from build123d import *

# Parameters (mm, degrees)
SKETCH1_W           = 27.7876
SKETCH1_H           = 4.572
CUT_EXTRUDE1_DEPTH  = 40.562666891
CUT_EXTRUDE2_DEPTH  = 40.562666891
CUT_EXTRUDE3_DEPTH  = 40.562666891
CUT_EXTRUDE4_DEPTH  = 40.562666891
CUT_EXTRUDE5_DEPTH  = 40.530803878
CUT_EXTRUDE6_DEPTH  = 40.530803878
SKETCH8_R           = 14.2875
BOSS_EXTRUDE1_DEPTH = 0.889
SKETCH9_R           = 12.9794
BOSS_EXTRUDE2_DEPTH = 0.8128
BOSS_EXTRUDE2_TAPER = 45
SKETCH10_R          = 12.1666
BOSS_EXTRUDE3_DEPTH = 18.2372
BOSS_EXTRUDE4_START = 0.889
SKETCH11_R          = 14.2875
BOSS_EXTRUDE4_DEPTH = 0.889
CUT_EXTRUDE7_DEPTH  = 47.764743892
SKETCH13_W          = 2.5908
SKETCH13_H          = 4.572
SKETCH14_W          = 2.5908
SKETCH14_H          = 4.572
SKETCH15_W          = 2.5908
SKETCH15_H          = 4.572
SKETCH16_W          = 2.5908
SKETCH16_H          = 4.572
SKETCH17_W          = 2.5908
SKETCH17_H          = 4.572
SKETCH18_W          = 2.5908
SKETCH18_H          = 4.572
CHAMFER1_SIZE       = 0.254
FILLET1_R           = 0.127
FILLET2_R           = 0.7874
SKETCH19_R          = 9.350419414
BOSS_EXTRUDE7_DEPTH = 25.4


with BuildPart() as part:
    # Sketch1 → Revolve1 (revolve)
    with BuildSketch(Plane.XY, mode=Mode.PRIVATE) as revolve1_sk:
        with Locations((13.8938, 3.175)):
            Rectangle(SKETCH1_W, SKETCH1_H)
    revolve(revolve1_sk.sketch.rotate(Axis((0, 5.461, 0), (0, -1, 0)), 270), axis=Axis((0, 5.461, 0), (0, -1, 0)))

    # Sketch2 → Cut-Extrude1 (cut, through all)
    with BuildSketch(Plane.XZ.offset(-0.889)):
        with BuildLine():
            Line((-27.742216161, -1.5875), (-25.859959008, -1.5875))
            ThreePointArc((-25.859959008, -1.5875), (-26.4033, 0), (-25.859959008, 1.5875))
            Line((-25.859959008, 1.5875), (-27.742216161, 1.5875))
            ThreePointArc((-27.742216161, 1.5875), (-27.7876, 0), (-27.742216161, -1.5875))
        make_face()
    extrude(amount=-CUT_EXTRUDE1_DEPTH, mode=Mode.SUBTRACT)

    # Sketch3 → Cut-Extrude2 (cut, through all)
    with BuildSketch(Plane.XZ.offset(-0.889)):
        with BuildLine():
            Line((-15.245923409, 23.231713952), (-14.304794833, 21.601631442))
            ThreePointArc((-14.304794833, 21.601631442), (-13.20165, 22.865928544), (-11.555164176, 23.189131442))
            Line((-11.555164176, 23.189131442), (-12.496292752, 24.819213952))
            ThreePointArc((-12.496292752, 24.819213952), (-13.8938, 24.06476751), (-15.245923409, 23.231713952))
        make_face()
    extrude(amount=-CUT_EXTRUDE2_DEPTH, mode=Mode.SUBTRACT)

    # Sketch4 → Cut-Extrude3 (cut, through all)
    with BuildSketch(Plane.XZ.offset(-0.889)):
        with BuildLine():
            Line((12.496292752, 24.819213952), (11.555164176, 23.189131442))
            ThreePointArc((11.555164176, 23.189131442), (13.20165, 22.865928544), (14.304794833, 21.601631442))
            Line((14.304794833, 21.601631442), (15.245923409, 23.231713952))
            ThreePointArc((15.245923409, 23.231713952), (13.8938, 24.06476751), (12.496292752, 24.819213952))
        make_face()
    extrude(amount=-CUT_EXTRUDE3_DEPTH, mode=Mode.SUBTRACT)

    # Sketch5 → Cut-Extrude4 (cut, through all)
    with BuildSketch(Plane.XZ.offset(-0.889)):
        with BuildLine():
            Line((27.742216161, 1.5875), (25.859959008, 1.5875))
            ThreePointArc((25.859959008, 1.5875), (26.4033, 0), (25.859959008, -1.5875))
            Line((25.859959008, -1.5875), (27.742216161, -1.5875))
            ThreePointArc((27.742216161, -1.5875), (27.7876, 0), (27.742216161, 1.5875))
        make_face()
    extrude(amount=-CUT_EXTRUDE4_DEPTH, mode=Mode.SUBTRACT)

    # Sketch6 → Cut-Extrude5 (cut, through all)
    with BuildSketch(Plane.XZ.offset(-0.889)):
        with BuildLine():
            Line((15.245923409, -23.231713952), (14.304794833, -21.601631442))
            ThreePointArc((14.304794833, -21.601631442), (13.20165, -22.865928544), (11.555164176, -23.189131442))
            Line((11.555164176, -23.189131442), (12.496292752, -24.819213952))
            ThreePointArc((12.496292752, -24.819213952), (13.8938, -24.06476751), (15.245923409, -23.231713952))
        make_face()
    extrude(amount=-CUT_EXTRUDE5_DEPTH, mode=Mode.SUBTRACT)

    # Sketch7 → Cut-Extrude6 (cut, through all)
    with BuildSketch(Plane.XZ.offset(-0.889)):
        with BuildLine():
            Line((-12.496292752, -24.819213952), (-11.555164176, -23.189131442))
            ThreePointArc((-11.555164176, -23.189131442), (-13.20165, -22.865928544), (-14.304794833, -21.601631442))
            Line((-14.304794833, -21.601631442), (-15.245923409, -23.231713952))
            ThreePointArc((-15.245923409, -23.231713952), (-13.8938, -24.06476751), (-12.496292752, -24.819213952))
        make_face()
    extrude(amount=-CUT_EXTRUDE6_DEPTH, mode=Mode.SUBTRACT)

    # Sketch8 → Boss-Extrude1 (add)
    with BuildSketch(Plane(origin=(0, 5.461, 0), x_dir=(-1, 0, 0), z_dir=(0, 1, 0))):
        with Locations(Location((0, 0, 0), (0, 0, 90))):
            Circle(SKETCH8_R)
    extrude(amount=BOSS_EXTRUDE1_DEPTH)

    # Sketch9 → Boss-Extrude2 (add)
    with BuildSketch(Plane(origin=(0, 6.35, 0), x_dir=(-1, 0, 0), z_dir=(0, 1, 0))):
        Circle(SKETCH9_R)
    extrude(amount=BOSS_EXTRUDE2_DEPTH, taper=BOSS_EXTRUDE2_TAPER)

    # Sketch10 → Boss-Extrude3 (add)
    with BuildSketch(Plane(origin=(0, 7.1628, 0), x_dir=(-1, 0, 0), z_dir=(0, 1, 0))):
        with Locations(Location((0, 0, 0), (0, 0, 90))):
            Circle(SKETCH10_R)
    extrude(amount=BOSS_EXTRUDE3_DEPTH)

    # Sketch11 → Boss-Extrude4 (add)
    with BuildSketch(Plane.XZ.offset(-0.889).offset(BOSS_EXTRUDE4_START)):
        with Locations(Location((0, 0, 0), (0, 0, 90))):
            Circle(SKETCH11_R)
    extrude(amount=-BOSS_EXTRUDE4_DEPTH)

    # Sketch12 → Cut-Extrude7 (cut, through all)
    with BuildSketch(Plane.XZ):
        with BuildLine():
            Line((-8.0518, -1.65735), (-6.248228986, -1.65735))
            ThreePointArc((-6.248228986, -1.65735), (0, -6.4643), (6.248228986, -1.65735))
            Line((6.248228986, -1.65735), (8.0518, -1.65735))
            Line((8.0518, -1.65735), (8.0518, 1.65735))
            Line((8.0518, 1.65735), (6.248228986, 1.65735))
            ThreePointArc((6.248228986, 1.65735), (0, 6.4643), (-6.248228986, 1.65735))
            Line((-6.248228986, 1.65735), (-8.0518, 1.65735))
            Line((-8.0518, 1.65735), (-8.0518, -1.65735))
        make_face()
    extrude(amount=-CUT_EXTRUDE7_DEPTH, mode=Mode.SUBTRACT)

    # Sketch13 → Cut-Revolve1 (revolve, cut)
    with BuildSketch(Plane.XY):
        with Locations((-22.5171, 3.175)):
            Rectangle(SKETCH13_W, SKETCH13_H)
    revolve(axis=Axis((-23.8125, 5.461, 0), (0, -1, 0)), mode=Mode.SUBTRACT)

    # Sketch14 → Cut-Revolve2 (revolve, cut)
    with BuildSketch(Plane(origin=(0, 0, 20.622229928), x_dir=(-1, 0, 0), z_dir=(0, 0, -1))):
        with Locations((10.61085, 3.175)):
            Rectangle(SKETCH14_W, SKETCH14_H)
    revolve(axis=Axis((-11.90625, 0.889, 20.622229928), (0, 1, 0)), mode=Mode.SUBTRACT)

    # Sketch15 → Cut-Revolve3 (revolve, cut)
    with BuildSketch(Plane(origin=(0, 0, 20.622229928), x_dir=(-1, 0, 0), z_dir=(0, 0, -1))):
        with Locations((-13.20165, 3.175)):
            Rectangle(SKETCH15_W, SKETCH15_H)
    revolve(axis=Axis((11.90625, 0.889, 20.622229928), (0, 1, 0)), mode=Mode.SUBTRACT)

    # Sketch16 → Cut-Revolve4 (revolve, cut)
    with BuildSketch(Plane.XY):
        with Locations((25.1079, 3.175)):
            Rectangle(SKETCH16_W, SKETCH16_H)
    revolve(axis=Axis((23.8125, 5.461, 0), (0, -1, 0)), mode=Mode.SUBTRACT)

    # Sketch17 → Cut-Revolve5 (revolve, cut)
    with BuildSketch(Plane.XY.offset(-20.622229928)):
        with Locations((13.20165, 3.175)):
            Rectangle(SKETCH17_W, SKETCH17_H)
    revolve(axis=Axis((11.90625, 5.461, -20.622229928), (0, -1, 0)), mode=Mode.SUBTRACT)

    # Sketch18 → Cut-Revolve6 (revolve, cut)
    with BuildSketch(Plane.XY.offset(-20.622229928)):
        with Locations((-10.61085, 3.175)):
            Rectangle(SKETCH18_W, SKETCH18_H)
    revolve(axis=Axis((-11.90625, 5.461, -20.622229928), (0, -1, 0)), mode=Mode.SUBTRACT)

    # Chamfer1
    chamfer1_edges = [part.edges().sort_by_distance(p)[0] for p in [
        (0, 6.35, -14.2875),
        (0, 25.4, -12.1666),
        (0, 0, -14.2875),
        (0, 25.4, 6.4643),
        (0, 25.4, -6.4643),
        (0, 0, -6.4643),
        (0, 0, 6.4643),
    ]]
    chamfer(chamfer1_edges, length=CHAMFER1_SIZE)

    # Fillet1
    fillet1_edges = [part.edges().sort_by_distance(p)[0] for p in [
        (-6.248228986, 12.7, 1.65735),
        (-8.0518, 12.7, 1.65735),
        (-8.0518, 12.7, -1.65735),
        (6.248228986, 12.7, 1.65735),
        (-6.248228986, 12.7, -1.65735),
        (8.0518, 12.7, 1.65735),
        (8.0518, 12.7, -1.65735),
        (6.248228986, 12.7, -1.65735),
    ]]
    fillet(fillet1_edges, radius=FILLET1_R)

    # Fillet2
    fillet2_edges = [part.edges().sort_by_distance(p)[0] for p in [
        (-27.742216161, 3.175, -1.5875),
        (-27.742216161, 3.175, 1.5875),
        (-25.859959008, 3.175, 1.5875),
        (-25.859959008, 3.175, -1.5875),
        (-15.245923409, 3.175, 23.231713952),
        (-12.496292752, 3.175, 24.819213952),
        (-11.555164176, 3.175, 23.189131442),
        (-14.304794833, 3.175, 21.601631442),
        (12.496292752, 3.175, 24.819213952),
        (15.245923409, 3.175, 23.231713952),
        (14.304794833, 3.175, 21.601631442),
        (11.555164176, 3.175, 23.189131442),
        (27.742216161, 3.175, 1.5875),
        (27.742216161, 3.175, -1.5875),
        (25.859959008, 3.175, -1.5875),
        (25.859959008, 3.175, 1.5875),
        (15.245923409, 3.175, -23.231713952),
        (12.496292752, 3.175, -24.819213952),
        (11.555164176, 3.175, -23.189131442),
        (14.304794833, 3.175, -21.601631442),
        (-12.496292752, 3.175, -24.819213952),
        (-15.245923409, 3.175, -23.231713952),
        (-14.304794833, 3.175, -21.601631442),
        (-11.555164176, 3.175, -23.189131442),
    ]]
    fillet(fillet2_edges, radius=FILLET2_R)

    # Sketch19 → Boss-Extrude7 (add)
    with BuildSketch(Plane(origin=(0, 25.4, 0), x_dir=(1, 0, 0), z_dir=(0, 1, 0))):
        Circle(SKETCH19_R)
    extrude(amount=-BOSS_EXTRUDE7_DEPTH)


solid = part.part
Part model, mm, in its own coordinate system. A direction names the side the tool comes from. Coordinates: 2 decimals unless noted, no trailing zeros. Order: outer loops, then holes, each group sorted by start corner. A loop starts at its lowest first (then second) coordinate and runs counter-clockwise, first axis right, second up. Notation, with made-up numbers: (52, 50.5) - (102, 50.5) arc R4 ccw to (102, 55.5) - close; hole circle Ø10 at (63.25, 1.5). An arc over 180 degrees is marked (long way). Use CSV: the item, a comma, the result in double quotes.
Item 1: 3-axis set-ups, long thin cutter, end or side, ignore diameter. For faces 5 (the face through (-0.628, 0.567, -14.274)), 6 (the face through (-24.149, 3.207, -13.747)), 7 (the face through (13, 5.461, -7)): which of +Z, -Z, +X, -X, +Y, -Y reach the whole face in a straight line?
Solved:
face 5,"-Y"
face 6,"-Z, -X, +Y, -Y"
face 7,"+Y"
Item 2: Drop flat-ended pins along their axis: P1, Ø8, axis at x = 12.5, y = 15.5, coming from the -Z side; P2, Ø6.5, axis at x = -11.91, z = 20.62, coming from the +Y side; P3, Ø1.5, axis at y = 18.5, z = -0.5, coming from the +X side. Give the stop position or say it passes through.
Solved:
P1,"stops at z = -8.7"
P2,"stops at y = 5.46"
P3,"stops at x = 12.17"
Item 3: Mould opens along X. For faces 1 (the face through (-9.3, 6.35, 9.3)), 2 (the face through (23.98, 3.21, -14.04)), 3 (the face through (10.686, 3.207, -18.337)), 4 (the face through (10.686, 3.207, 18.337)) say: +X half, -X half, draft (parallel to the pull), parting line (faces both ways), or undercut.
Solved:
face 1,"draft"
face 2,"+X half"
face 3,"undercut"
face 4,"undercut"
Item 4: Saw through at A-A on x = 0. Give the cut face in (y, z).
Solved:
outline,"(0, -14.03) - (0.25, -14.29) - (0.89, -14.29) - (0.89, -27.79) - (5.46, -27.79) - (5.46, -14.29) - (6.1, -14.29) - (6.35, -14.03) - (6.35, -12.98) - (7.16, -12.17) - (25.15, -12.17) - (25.4, -11.91) - (25.4, 11.91) - (25.15, 12.17) - (7.16, 12.17) - (6.35, 12.98) - (6.35, 14.03) - (6.1, 14.29) - (5.46, 14.29) - (5.46, 27.79) - (0.89, 27.79) - (0.89, 14.29) - (0.25, 14.29) - (0, 14.03) - close"
Item 5: Saw through at B-B on y = 22.5. Give the cut face in (x, z).
Solved:
outline,"circle Ø24.33 at (0, 0)"
Item 6: Probe probe 1 along X at (y, z) = (2, 22) (3 decimals); probe 2 along Y at (x, z) = (-5.5, -21); probe 3 along Z at (x, y) = (-10, 14.75). List the from-to ranges inside material, lowest first.
Solved:
probe 1,"x = -16.975 to -14.535, -9.712 to 9.712, 14.535 to 16.975"
probe 2,"y = 0.89 to 5.46"
probe 3,"z = -6.93 to 6.93"
